Design review of the part shown in the three views and the two pictorial views. Dimensions are in mm from the part's minimum x, y and z. A direction names the side the tool comes from. Give positions to 0.01 mm unless a question says otherwise; leave off trailing zeros. Write each loop counter-clockwise with the first axis right and the second up, starting at its lowest first coordinate (ties: lowest second). Pieces come first, ordered by that corner, then holes. Notation, with made-up numbers: (84, 72) -> (108, 72) arc R10 ccw to (108, 79) -> close; hole circle Ø4 at (16.5, 65). An arc over 180 degrees is marked (long way). Use CSV: the item, a comma, the result in double quotes.
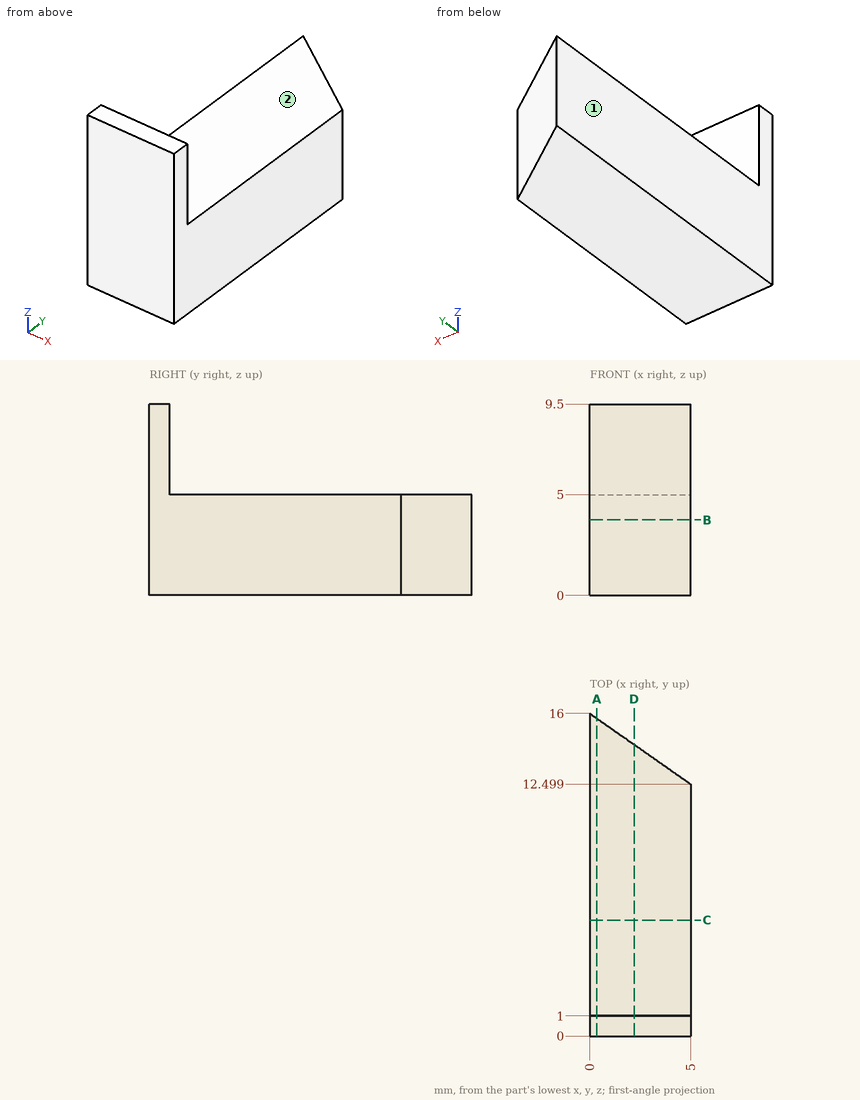
Q1. To check wall thickness, follow probe 1 along Z at (x, y) = (0.4, 11.5); probe 2 along Y at (x, z) = (2.95, 6.75); probe 3 along Y at (x, z) = (0.95, 2.75). State the ranges of each line that lie inside material, in increasing order.
Derived:
probe 1,"z = 0 to 5"
probe 2,"y = 0 to 1"
probe 3,"y = 0 to 15.33"
Q2. Consider section D-D (x = 2.2). Write out the cut boundary in (y, z), then the cut area to 3 significant figures.
Derived:
outline,"(0, 0) -> (14.46, 0) -> (14.46, 5) -> (1, 5) -> (1, 9.5) -> (0, 9.5) -> close"
area,"76.8 mm2"
Q3. Insertion check: pin 1 (5 mm diameter, centred on y = 3.5, z = 6.5, fed in from -X). The pin has a flat end and moves straight along its axis. Give the tip position at first contact, or say it passes through.
Derived:
pin 1,"stops at x = 0"
Q4. Machinability: for the marked faces 1 and 2, which of the approach directions +Z, -Z, +X, -X, +Y, -Y give a long, thin tool a straight path to every point of the face, cutting with its end or side? Answer none if there is none.
Derived:
face 1,"+Z, -Z, -X, +Y, -Y"
face 2,"+Z, +X, -X, +Y"
Q5. Consider section A-A (x = 0.35). Write out the cut boundary in (y, z) (3 decimals), then the cut area to 3 significant figures.
Derived:
outline,"(0, 0) -> (15.755, 0) -> (15.755, 5) -> (1, 5) -> (1, 9.5) -> (0, 9.5) -> close"
area,"83.3 mm2"
Q6. Consider section C-C (y = 5.75). Write out the cut boundary in (x, z).
Derived:
outline,"(0, 0) -> (5, 0) -> (5, 5) -> (0, 5) -> close"
Q7. Consider section B-B (z = 3.75). Write out the cut boundary in (x, y).
Derived:
outline,"(0, 0) -> (5, 0) -> (5, 12.5) -> (0, 16) -> close"
